```python
from build123d import *

# Parameters (mm, degrees)
ESQUISSE1_W      = 187
ESQUISSE1_H      = 96
ESQUISSE1_R      = 1.5
EXTRUSION1_DEPTH = 3
ESQUISSE2_W      = 55
ESQUISSE2_H      = 5
EXTRUSION2_DEPTH = 10
ESQUISSE4_W      = 10
ESQUISSE4_H      = 5
EXTRUSION4_DEPTH = 10


with BuildPart() as part:
    # Esquisse1 → Extrusion1 (new body)
    with BuildSketch(Plane(origin=(0, 0, 0), x_dir=(1, 0, 0), z_dir=(0, 1, 0))):
        with Locations((93.5, 48)):
            Rectangle(ESQUISSE1_W, ESQUISSE1_H)
        with Locations((5, 91)):
            Circle(ESQUISSE1_R, mode=Mode.SUBTRACT)
        with Locations((182, 91)):
            Circle(ESQUISSE1_R, mode=Mode.SUBTRACT)
        with Locations((182, 5)):
            Circle(ESQUISSE1_R, mode=Mode.SUBTRACT)
        with Locations((5, 5)):
            Circle(ESQUISSE1_R, mode=Mode.SUBTRACT)
    extrude(amount=EXTRUSION1_DEPTH)

    # Esquisse2 → Extrusion2 (add)
    with BuildSketch(Plane(origin=(0, 3, 0), x_dir=(1, 0, 0), z_dir=(0, 1, 0))):
        with Locations((93.5, 83)):
            Rectangle(ESQUISSE2_W, ESQUISSE2_H)
        with Locations((93.5, 13)):
            Rectangle(ESQUISSE2_W, ESQUISSE2_H)
    extrude(amount=EXTRUSION2_DEPTH)

    # Esquisse4 → Extrusion4 (add)
    with BuildSketch(Plane(origin=(0, 3, 0), x_dir=(1, 0, 0), z_dir=(0, 1, 0))):
        with Locations((165.295070297, 63.362289653)):
            Rectangle(ESQUISSE4_W, ESQUISSE4_H)
        with Locations((13.593769781, 63.362289653)):
            Rectangle(ESQUISSE4_W, ESQUISSE4_H)
        with Locations((13.593769781, 38.362289653)):
            Rectangle(ESQUISSE4_W, ESQUISSE4_H)
        with Locations((13.593769781, 25.862289653)):
            Rectangle(ESQUISSE4_W, ESQUISSE4_H)
        with Locations((13.593769781, 50.862289653)):
            Rectangle(ESQUISSE4_W, ESQUISSE4_H)
        with Locations((165.295070297, 38.362289653)):
            Rectangle(ESQUISSE4_W, ESQUISSE4_H)
        with Locations((165.295070297, 25.862289653)):
            Rectangle(ESQUISSE4_W, ESQUISSE4_H)
        with Locations((165.295070297, 50.862289653)):
            Rectangle(ESQUISSE4_W, ESQUISSE4_H)
    extrude(amount=EXTRUSION4_DEPTH)


solid = part.part
```
Work out the finished part from the listing and answer in its coordinate system (mm). A direction names the side the tool comes from. Give positions to 0.01 mm unless a question says otherwise; leave off trailing zeros. Loops run counter-clockwise (first coordinate to the right, second up) from the corner with the lowest first, then second, coordinate; pieces in that order, holes last. Notation, with made-up numbers: (16, 30) -> (62, 30) arc R18 cw to (62, 52) -> close; hole circle Ø1 at (-37.75, 75). An arc over 180 degrees is marked (long way). Use CSV: the item, a comma, the result in double quotes.
1. Straight lines are drawn through the part: line 1 (X direction, y = 1.3, z = -91); line 2 (Z direction, x = 167, y = 6.75); line 3 (Z direction, x = 182, y = 1.65). For each, find the intervals that lie inside material, in ascending order.
Found:
line 1,"0 to 3.5, 6.5 to 180.5, 183.5 to 187"
line 2,"-65.86 to -60.86, -53.36 to -48.36, -40.86 to -35.86, -28.36 to -23.36"
line 3,"-96 to -92.5, -89.5 to -6.5, -3.5 to 0"
2. The part is cut by section B-B (y = 10.75). State how many separate pieces and enclosed holes the cut face has, then the cut area to 3 significant figures.
Found:
separate pieces,"10"
enclosed holes,"0"
area,"950 mm^2"
3. The part is cut by section D-D (x = 168). Write down the section's boundary in (y, z).
Found:
outline,"(0, -96) -> (3, -96) -> (3, -65.86) -> (13, -65.86) -> (13, -60.86) -> (3, -60.86) -> (3, -53.36) -> (13, -53.36) -> (13, -48.36) -> (3, -48.36) -> (3, -40.86) -> (13, -40.86) -> (13, -35.86) -> (3, -35.86) -> (3, -28.36) -> (13, -28.36) -> (13, -23.36) -> (3, -23.36) -> (3, 0) -> (0, 0) -> close"
4. The part is cut by section A-A (x = 99). Write down the section's boundary in (y, z).
Found:
outline,"(0, -96) -> (3, -96) -> (3, -85.5) -> (13, -85.5) -> (13, -80.5) -> (3, -80.5) -> (3, -15.5) -> (13, -15.5) -> (13, -10.5) -> (3, -10.5) -> (3, 0) -> (0, 0) -> close"
5. The mould has two halves that part along X. Classify faces 5 (the flat face through (170.295, 8, -38)), 6 (the flat face through (160.295, 8, -63)), 7 (the flat face through (14, 13, -51)): +X half, -X half, draft (parallel to the pull), parting line (faces both ways), or undercut.
Found:
face 5,"+X half"
face 6,"undercut"
face 7,"draft"
6. A tool of negligible diameter and unlimited length cuts with its end or side. For faces 1 (the flat face through (93, 13, -13)), 2 (the flat face through (8.594, 8, -26)), 3 (the flat face through (165, 8, -53.362)), 4 (the flat face through (18.594, 8, -51)), from which of +Z, -Z, +X, -X, +Y, -Y can it reach the whole face along a straight path? Write none if from no direction.
Found:
face 1,"+Z, -Z, +X, -X, +Y"
face 2,"+Z, -Z, -X, +Y"
face 3,"+X, -X, +Y"
face 4,"+Z, -Z, +Y"
7. The part is cut by section C-C (z = -69). Write down the section's boundary in (x, y), then the cut area to 3 significant figures.
Found:
outline,"(0, 0) -> (187, 0) -> (187, 3) -> (0, 3) -> close"
area,"561 mm^2"
8. Flat-ended cylindrical pins translate along their axes: pin 1 Ø3 at (x, y) = (14.5, 9) entering from -Z; pin 2 Ø2.5 at (y, z) = (9.5, -83.5) entering from +X; pin 3 Ø4 at (y, z) = (7, -25) entering from +X. Find the tip coordinate at first contact, or state that the pin passes through.
Found:
pin 1,"z = -65.86"
pin 2,"x = 121"
pin 3,"x = 170.3"
